The listing builds one solid part. Answer for the finished solid, in the listing's coordinates (mm). A direction names the side the tool comes from. Coordinates: 2 decimals unless noted, no trailing zeros. Loops run counter-clockwise (first coordinate to the right, second up) from the corner with the lowest first, then second, coordinate; pieces in that order, holes last. Notation, with made-up numbers: (-40, 79.25) - (-25, 79.25) arc R7 cw to (-25, 90.25) - close; hole circle Ø11 at (54, -32.5). An arc over 180 degrees is marked (long way). Use one line per item in the form item = value. Start each with the question number.
```python
from build123d import *

# Parameters (mm, degrees)
F0_W     = 23.75
F0_H     = 22
F1_DEPTH = 15
F2_DEPTH = 2
F3_DEPTH = 2


with BuildPart() as f1:
    # F0 (on Top) → F1 (new body)
    with BuildSketch(Plane.XY):
        Polygon((-34.75, -9.78861), (-34.75, -11.78861), (69.25, -11.78861), (69.25, 2.46139), (94.75, 2.46139), (94.75, 12.21139), (104.25, 12.21139), (104.25, 12.13003), (105.9946, 12.13003), (105.9946, 18.31139), (104.25, 18.31139), (71.25, 18.31139), (71.25, 24.96139), (71.25, 26.71139), (-26.958708, 26.71139), (-34.75, 26.71139), (-34.75, 24.96139), (-34.75, 13.96139), (-34.75, 12.21139), align=None)
        Polygon((-32.75, -9.78861), (-32.75, 12.21139), (-19.336179, 12.21139), (-9, 12.21139), (-9, -9.78861), (-19.336179, -9.78861), align=None, mode=Mode.SUBTRACT)
        with Locations((4.625, 1.21139)):
            Rectangle(F0_W, F0_H, mode=Mode.SUBTRACT)
        with Locations((30.125, 1.21139)):
            Rectangle(F0_W, F0_H, mode=Mode.SUBTRACT)
        with Locations((55.625, 1.21139)):
            Rectangle(F0_W, F0_H, mode=Mode.SUBTRACT)
        Polygon((0, 13.96139), (-33, 13.96139), (-33, 24.96139), (-26.958708, 24.96139), (0, 24.96139), align=None, mode=Mode.SUBTRACT)
        Polygon((1.75, 13.96139), (1.75, 24.96139), (24.202205, 24.96139), (32.815558, 24.96139), (34.75, 24.96139), (34.75, 13.96139), (32.815558, 13.96139), (24.202205, 13.96139), align=None, mode=Mode.SUBTRACT)
        Polygon((69.25, 4.21139), (69.25, 12.21139), (87.25, 12.21139), (93, 12.21139), (93, 4.21139), align=None, mode=Mode.SUBTRACT)
        Polygon((102.25, 13.96139), (71.25, 13.96139), (71.25, 16.56139), (104.2446, 16.56139), (104.2446, 13.96139), align=None, mode=Mode.SUBTRACT)
        Polygon((36.5, 13.96139), (36.5, 24.96139), (69.5, 24.96139), (69.5, 18.31139), (69.5, 16.56139), (69.5, 13.96139), (69.25, 13.96139), (63.25, 13.96139), align=None, mode=Mode.SUBTRACT)
    extrude(amount=F1_DEPTH)

    # F0 (on Top) → F2 (join)
    with BuildSketch(Plane.XY):
        Polygon((-34.75, -9.78861), (-34.75, -11.78861), (69.25, -11.78861), (69.25, 2.46139), (94.75, 2.46139), (94.75, 12.21139), (104.25, 12.21139), (104.25, 12.13003), (105.9946, 12.13003), (105.9946, 18.31139), (104.25, 18.31139), (71.25, 18.31139), (71.25, 24.96139), (71.25, 26.71139), (-26.958708, 26.71139), (-34.75, 26.71139), (-34.75, 24.96139), (-34.75, 13.96139), (-34.75, 12.21139), align=None)
        Polygon((-32.75, -9.78861), (-32.75, 12.21139), (-19.336179, 12.21139), (-9, 12.21139), (-9, -9.78861), (-19.336179, -9.78861), align=None, mode=Mode.SUBTRACT)
        with Locations((4.625, 1.21139)):
            Rectangle(F0_W, F0_H, mode=Mode.SUBTRACT)
        with Locations((30.125, 1.21139)):
            Rectangle(F0_W, F0_H, mode=Mode.SUBTRACT)
        with Locations((55.625, 1.21139)):
            Rectangle(F0_W, F0_H, mode=Mode.SUBTRACT)
        Polygon((0, 13.96139), (-33, 13.96139), (-33, 24.96139), (-26.958708, 24.96139), (0, 24.96139), align=None, mode=Mode.SUBTRACT)
        Polygon((1.75, 13.96139), (1.75, 24.96139), (24.202205, 24.96139), (32.815558, 24.96139), (34.75, 24.96139), (34.75, 13.96139), (32.815558, 13.96139), (24.202205, 13.96139), align=None, mode=Mode.SUBTRACT)
        Polygon((69.25, 4.21139), (69.25, 12.21139), (87.25, 12.21139), (93, 12.21139), (93, 4.21139), align=None, mode=Mode.SUBTRACT)
        Polygon((102.25, 13.96139), (71.25, 13.96139), (71.25, 16.56139), (104.2446, 16.56139), (104.2446, 13.96139), align=None, mode=Mode.SUBTRACT)
        Polygon((36.5, 13.96139), (36.5, 24.96139), (69.5, 24.96139), (69.5, 18.31139), (69.5, 16.56139), (69.5, 13.96139), (69.25, 13.96139), (63.25, 13.96139), align=None, mode=Mode.SUBTRACT)
        Polygon((71.25, 16.56139), (71.25, 13.96139), (102.25, 13.96139), (104.2446, 13.96139), (104.2446, 16.56139), align=None)
    extrude(amount=F2_DEPTH)

    # F0 (on Top) → F3 (join)
    with BuildSketch(Plane.XY):
        Polygon((69.5, 24.96139), (36.5, 24.96139), (36.5, 13.96139), (63.25, 13.96139), (69.25, 13.96139), (69.5, 13.96139), (69.5, 16.56139), (69.5, 18.31139), align=None)
        with Locations((55.625, 1.21139)):
            Rectangle(F0_W, F0_H)
        Polygon((87.25, 12.21139), (69.25, 12.21139), (69.25, 4.21139), (93, 4.21139), (93, 12.21139), align=None)
        with Locations((30.125, 1.21139)):
            Rectangle(F0_W, F0_H)
        Polygon((24.202205, 24.96139), (1.75, 24.96139), (1.75, 13.96139), (24.202205, 13.96139), (32.815558, 13.96139), (34.75, 13.96139), (34.75, 24.96139), (32.815558, 24.96139), align=None)
        with Locations((4.625, 1.21139)):
            Rectangle(F0_W, F0_H)
        Polygon((-33, 24.96139), (-33, 13.96139), (0, 13.96139), (0, 24.96139), (-26.958708, 24.96139), align=None)
        Polygon((-19.336179, 12.21139), (-32.75, 12.21139), (-32.75, -9.78861), (-19.336179, -9.78861), (-9, -9.78861), (-9, 12.21139), align=None)
        Polygon((71.25, 16.56139), (71.25, 13.96139), (102.25, 13.96139), (104.2446, 13.96139), (104.2446, 16.56139), align=None)
    extrude(amount=F3_DEPTH)


solid = f1.part
```
(1) Determine the mould class of faces 1 (the face through (81, 12.211, 8)), 2 (the face through (-34.75, 8, 7)), 3 (the face through (17, -11.789, 7)) for opening direction X: +X half, -X half, draft (parallel to the pull), parting line (faces both ways), or undercut.
(2) A cutting plane is placed at D-D (x = 89.5). Determine the outline of the cut face in (y, z).
(3) For faces 4 (the face through (19, 26.711, 7)), 5 (the face through (0, 20, 8)), determine the directions among +Z, -Z, +X, -X, +Y, -Y from which every point of the face is accessible in a straight line to the end or side of a thin tool.
(4) A cutting plane is placed at C-C (z = 8). State how many separate pieces and enclosed holes the cut face has, then the cut area to 3 significant figures.
(5) Each of these flat-tipped pins is pushed along its axis until it touches: pin 1 Ø3 at (x, y) = (54, 17.5) entering from +Z; pin 2 Ø1.5 at (y, z) = (8, 13.5) entering from +X; pin 3 Ø1.5 at (y, z) = (19.5, 1.5) entering from +X. Where does it stop, or does it pass through?
(6) A cutting plane is placed at B-B (y = -5). Determine the outline of the cut face in (x, z), then the cut area to 3 significant figures.
(7) Find the intervals of material crossed by probe 1 along X at (y, z) = (21, 8.75); probe 2 along Y at (x, z) = (-3, 10.5); probe 3 along X at (y, z) = (-4, 13), in increasing order. Write a range as from..to.
(8) A cutting plane is placed at A-A (x = 25). Determine the outline of the cut face in (y, z), then the cut area to 4 significant figures.
Evaluation:
q1.face_1 = undercut
q1.face_2 = -X half
q1.face_3 = draft
q2.outline = (2.46, 0) - (18.31, 0) - (18.31, 15) - (16.56, 15) - (16.56, 2) - (13.96, 2) - (13.96, 15) - (12.21, 15) - (12.21, 2) - (4.21, 2) - (4.21, 15) - (2.46, 15) - close
q3.face_4 = +Z, -Z, +X, -X, +Y
q3.face_5 = +Z
q4.separate_pieces = 1
q4.enclosed_holes = 9
q4.area = 1,040 mm^2
q5.pin_1 = 2
q5.pin_2 = 94.75
q5.pin_3 = 71.25
q6.outline = (-34.75, 0) - (69.25, 0) - (69.25, 15) - (67.5, 15) - (67.5, 2) - (43.75, 2) - (43.75, 15) - (42, 15) - (42, 2) - (18.25, 2) - (18.25, 15) - (16.5, 15) - (16.5, 2) - (-7.25, 2) - (-7.25, 15) - (-9, 15) - (-9, 2) - (-32.75, 2) - (-32.75, 15) - (-34.75, 15) - close
q6.area = 325 mm^2
q7.probe_1 = -34.75..-33, 0..1.75, 34.75..36.5, 69.5..71.25
q7.probe_2 = -11.79..-9.79, 12.21..13.96, 24.96..26.71
q7.probe_3 = -34.75..-32.75, -9..-7.25, 16.5..18.25, 42..43.75, 67.5..69.25
q8.outline = (-11.79, 0) - (26.71, 0) - (26.71, 15) - (24.96, 15) - (24.96, 2) - (13.96, 2) - (13.96, 15) - (12.21, 15) - (12.21, 2) - (-9.79, 2) - (-9.79, 15) - (-11.79, 15) - close
q8.area = 148.5 mm^2
